Geometry: final body of the model. Coordinates: model frame, mm. Face numbers are marked on the shaded views. Coordinates: 2 decimals unless noted, no trailing zeros. Order: outer loops, then holes, each group sorted by start corner. A loop starts at its lowest first (then second) coordinate and runs counter-clockwise, first axis right, second up. Notation, with made-up numbers: M 40.25,-21.75 L 50.25,-21.75 A34 ccw 50.25,10.25 Z; hole C -30.75,59.5 d5. An arc over 180 degrees is marked long. Write item = value, one per line.
from build123d import *

# Parameters (mm, degrees)
BASE_EXTRUDE_DEPTH = 3


with BuildPart() as part:
    # Sketch1 → Base-Extrude (new body)
    with BuildSketch(Plane.XY):
        with BuildLine():
            Line((195.167267959, -118.672665529), (198.339039248, -124.445885207))
            ThreePointArc((198.339039248, -124.445885207), (199.392796981, -123.370856688), (200.158445725, -122.07475728))
            Line((200.158445725, -122.07475728), (200.158445725, -62.170573778))
            ThreePointArc((200.158445725, -62.170573778), (199.392796981, -60.874474369), (198.339039248, -59.79944585))
            Line((198.339039248, -59.79944585), (195.167267959, -65.572665529))
            Line((195.167267959, -65.572665529), (192.537947509, -64.128133088))
            Line((192.537947509, -64.128133088), (195.771956334, -58.576419897))
            ThreePointArc((195.771956334, -58.576419897), (190.863435389, -59.561310884), (188.258458895, -63.836551882))
            Line((188.258458895, -63.836551882), (188.258458895, -71.172665529))
            Line((188.258458895, -71.172665529), (194.386873079, -71.172665529))
            Line((194.386873079, -71.172665529), (194.386873079, -74.172665529))
            Line((194.386873079, -74.172665529), (187.843216204, -74.172665529))
            ThreePointArc((187.843216204, -74.172665529), (178.389950643, -92.122665529), (187.843216204, -110.072665529))
            Line((187.843216204, -110.072665529), (194.386873079, -110.072665529))
            Line((194.386873079, -110.072665529), (194.386873079, -113.072665529))
            Line((194.386873079, -113.072665529), (188.258458895, -113.072665529))
            Line((188.258458895, -113.072665529), (188.258458895, -120.408779175))
            ThreePointArc((188.258458895, -120.408779175), (190.863435389, -124.684020173), (195.771956334, -125.66891116))
            Line((195.771956334, -125.66891116), (192.537947509, -120.117197969))
            Line((192.537947509, -120.117197969), (195.167267959, -118.672665529))
        make_face()
    extrude(amount=BASE_EXTRUDE_DEPTH)


solid = part.part
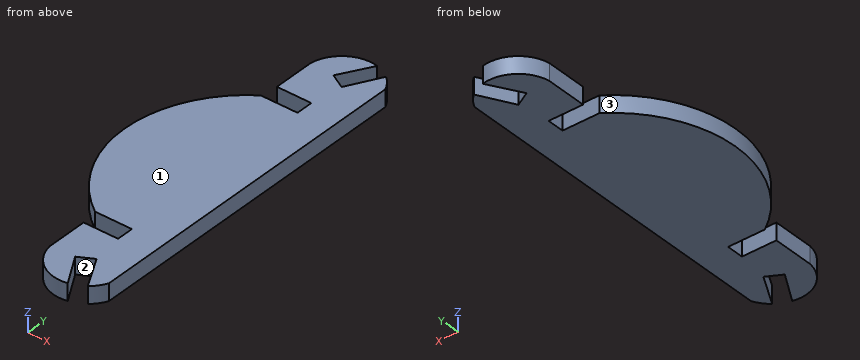
1) Section D-D, the plane x = 180. Return loops of the section in (y, z), and give its area (3 significant figures).
Numbers:
outline = M -100.34,0 L -83.91,0 L -83.91,3 L -100.34,3 Z
area = 49.3 mm²
2) Line query: L1, parallel to Y at x = 194, z = 1.6; L2, parallel to Y at x = 195.5, z = 1.7; L3, parallel to Y at x = 195.25, z = 0.3. Output: solid intervals per line, ascending.
Numbers:
L1 = -125.8 to -122.63, -119.31 to -113.07, -110.07 to -74.17, -71.17 to -64.93, -61.62 to -58.45
L2 = -125.72 to -125.2, -119.28 to -64.97, -59.04 to -58.52
L3 = -125.76 to -124.77, -118.82 to -65.42, -59.47 to -58.49
3) Section A-A, the plane x = 189.5. Return loops of the section in (y, z), and give its area (3 significant figures).
Numbers:
outline = M -123.38,0 L -113.07,0 L -113.07,3 L -123.38,3 Z; M -110.07,0 L -74.17,0 L -74.17,3 L -110.07,3 Z; M -71.17,0 L -60.86,0 L -60.86,3 L -71.17,3 Z
area = 170 mm²
4) Mould query, pull axis Y, two halves, no side actions, for the marked faces 1, 2 and 3. Classes: pulls with the +Y half, pulls with the -Y half, needs draft (parallel to the pull), parting line crosses it, or undercut.
Numbers:
face_1 = needs draft
face_2 = undercut
face_3 = parting line crosses it
5) Section B-B, the plane z = 1. Return loops of the section in (x, y).
Numbers:
outline = M 187.84,-110.07 L 194.39,-110.07 L 194.39,-113.07 L 188.26,-113.07 L 188.26,-120.41 A6.24 ccw 195.77,-125.67 L 192.54,-120.12 L 195.17,-118.67 L 198.34,-124.45 A6.24 ccw 200.16,-122.07 L 200.16,-62.17 A6.24 ccw 198.34,-59.8 L 195.17,-65.57 L 192.54,-64.13 L 195.77,-58.58 A6.24 ccw 188.26,-63.84 L 188.26,-71.17 L 194.39,-71.17 L 194.39,-74.17 L 187.84,-74.17 A21.77 ccw Z
6) Pin query (flat end, axial travel): pin 1 (0.9 mm diameter, centred on x = 190, z = 2, fed in from +Y); pin 2 (4 mm diameter, centred on x = 195, y = -78.5, fed in from -Z); pin 3 (1.5 mm diameter, centred on x = 192.5, z = 1.5, fed in from +Y); pin 4 (1.5 mm diameter, centred on x = 191.5, z = 2, fed in from -Y). Return the tip coordinate at first contact, or that it passes through.
Numbers:
pin_1 = -59.88
pin_2 = 0
pin_3 = -58.55
pin_4 = -125.41
7) Section C-C, the plane y = -79. Return loops of the section in (x, z).
Numbers:
outline = M 182.79,0 L 200.16,0 L 200.16,3 L 182.79,3 Z
